Build history of the part. All positions in model axes, mm. Face numbers are marked on the shaded views. A direction names the side the tool comes from. Round coordinates to 2 decimals unless told otherwise and drop trailing zeros. Write each loop counter-clockwise with the first axis right and the second up, starting at its lowest first coordinate (ties: lowest second). Pieces come first, ordered by that corner, then holes. Notation, with made-up numbers: (82.5, -13.75) -> (96.5, -13.75) arc R32 ccw to (96.5, 16.25) -> close; hole circle Ø5 at (23.5, 48). An arc over 180 degrees is marked (long way). Return JSON: item names as keys, results as strings.
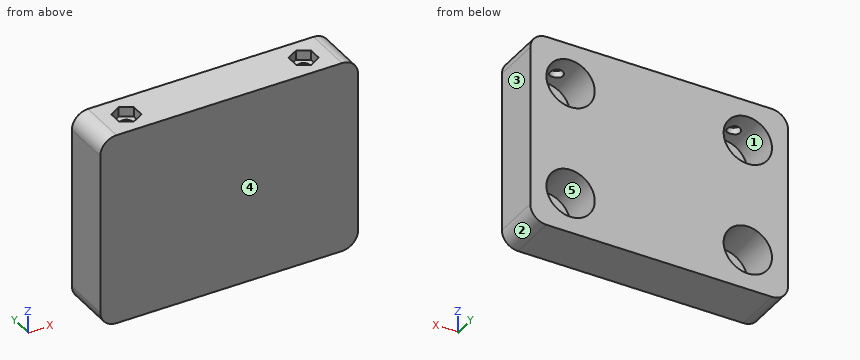
from build123d import *

# Parameters (mm, degrees)
F1_DEPTH = 15
F2_R     = 7.5
F3_DEPTH = 13
F4_R     = 2
F5_DEPTH = 6
F7_DEPTH = 3


with BuildPart() as f1:
    # F0 (on Front) → F1 (new body)
    with BuildSketch(Plane.XZ):
        with BuildLine():
            Line((-0.08701, 32.806785), (-70.08701, 32.806785))
            ThreePointArc((-70.08701, 32.806785), (-73.622544, 31.342318), (-75.08701, 27.806785))
            Line((-75.08701, 27.806785), (-75.08701, -22.193215))
            ThreePointArc((-75.08701, -22.193215), (-73.622544, -25.728749), (-70.08701, -27.193215))
            Line((-70.08701, -27.193215), (-0.08701, -27.193215))
            ThreePointArc((-0.08701, -27.193215), (3.448524, -25.728749), (4.91299, -22.193215))
            Line((4.91299, -22.193215), (4.91299, 27.806785))
            ThreePointArc((4.91299, 27.806785), (3.448524, 31.342318), (-0.08701, 32.806785))
        make_face()
    extrude(amount=F1_DEPTH)

    # F2 (on face) → F3 (cut)
    with BuildSketch(Plane(origin=(0, 0, 0), x_dir=(-1, 0, 0), z_dir=(0, 1, 0))):
        with Locations((7.58701, 20.306785)):
            Circle(F2_R)
        with Locations((62.58701, 20.306785)):
            Circle(F2_R)
        with Locations((62.58701, -14.693215)):
            Circle(F2_R)
        with Locations((7.58701, -14.693215)):
            Circle(F2_R)
    extrude(amount=-F3_DEPTH, mode=Mode.SUBTRACT)

    # F4 (on face) → F5 (cut)
    with BuildSketch(Plane.XY.offset(32.806785)):
        with Locations((-62.58701, -7.5)):
            Circle(F4_R)
        with Locations((-7.58701, -7.5)):
            Circle(F4_R)
    extrude(amount=-F5_DEPTH, mode=Mode.SUBTRACT)

    # F6 (on face) → F7 (cut)
    with BuildSketch(Plane.XY.offset(32.806785)):
        Polygon((-59.08701, -9.520726), (-59.08701, -5.479274), (-62.58701, -3.458548), (-66.08701, -5.479274), (-66.08701, -9.520726), (-62.58701, -11.541452), align=None)
        Polygon((-4.08701, -9.520726), (-4.08701, -5.479274), (-7.58701, -3.458548), (-11.08701, -5.479274), (-11.08701, -9.520726), (-7.58701, -11.541452), align=None)
    extrude(amount=-F7_DEPTH, mode=Mode.SUBTRACT)


solid = f1.part
Q1. Saw through at A-A on y = -7.5. List the corners of the cut face in (x, z).
Verdict:
{"outline": "(-75.09, -22.19) arc R5 ccw to (-70.09, -27.19) -> (-0.09, -27.19) arc R5 ccw to (4.91, -22.19) -> (4.91, 27.81) arc R5 ccw to (-0.09, 32.81) -> (-4.09, 32.81) -> (-4.09, 29.81) -> (-5.59, 29.81) -> (-5.59, 27.54) arc R7.5 cw (long way) to (-9.59, 27.54) -> (-9.59, 29.81) -> (-11.09, 29.81) -> (-11.09, 32.81) -> (-59.09, 32.81) -> (-59.09, 29.81) -> (-60.59, 29.81) -> (-60.59, 27.54) arc R7.5 cw (long way) to (-64.59, 27.54) -> (-64.59, 29.81) -> (-66.09, 29.81) -> (-66.09, 32.81) -> (-70.09, 32.81) arc R5 ccw to (-75.09, 27.81) -> close; hole circle Ø15 at (-62.59, -14.69); hole circle Ø15 at (-7.59, -14.69)"}
Q2. Saw through at B-B on x = -63.5. List the corners of the cut face in (y, z).
Verdict:
{"outline": "(-15, -27.19) -> (0, -27.19) -> (0, -22.14) -> (-13, -22.14) -> (-13, -7.25) -> (0, -7.25) -> (0, 12.86) -> (-13, 12.86) -> (-13, 27.75) -> (-9.28, 27.75) -> (-9.28, 29.81) -> (-11.01, 29.81) -> (-11.01, 32.81) -> (-15, 32.81) -> close; (-5.72, 27.75) -> (0, 27.75) -> (0, 32.81) -> (-3.99, 32.81) -> (-3.99, 29.81) -> (-5.72, 29.81) -> close"}
Q3. 3-axis set-ups, long thin cutter, end or side, ignore diameter. For the marked faces 1 and 2: which of +Z, -Z, +X, -X, +Y, -Y reach the whole face in a straight line?
Verdict:
{"face 1": "+Y", "face 2": "-Z, +X, +Y, -Y"}
Q4. Two-plate mould, pull along X, no slides. Class the marked faces 3, 4 and 5: +X half, -X half, draft (parallel to the pull), parting line (faces both ways), or undercut.
Verdict:
{"face 3": "+X half", "face 4": "draft", "face 5": "undercut"}
Q5. Pin check, flat tips, straight feed: pin 1 Ø0.9 at (y, z) = (-6.5, 31) entering from -X; pin 2 Ø12 at (x, z) = (-6.5, -12.5) entering from +Y; pin 3 Ø1.5 at (y, z) = (-8, 31) entering from +X; pin 4 Ø4.5 at (x, z) = (-65, 22) entering from +Y. Stop position of each tip, or through.
Verdict:
{"pin 1": "stops at x = -74.27", "pin 2": "stops at y = 0", "pin 3": "stops at x = 4.28", "pin 4": "stops at y = -13"}
Q6. Saw through at D-D on z = 25.5. List the corners of the cut face in (x, y), then the cut area to 3 significant figures.
Verdict:
{"outline": "(-75.09, -15) -> (4.91, -15) -> (4.91, 0) -> (-2.18, 0) -> (-2.18, -13) -> (-13, -13) -> (-13, 0) -> (-57.18, 0) -> (-57.18, -13) -> (-68, -13) -> (-68, 0) -> (-75.09, 0) -> close", "area": "919 mm²"}
Q7. Wall check: L1, parallel to Z at x = -65.5, y = -1.5; L2, parallel to X at y = -11, z = -20; L3, parallel to X at y = -7, z = 30.5. Give the ranges that are in metal, low to high.
Verdict:
{"L1": "z = -27.19 to -21.6, -7.78 to 13.4, 27.22 to 32.81", "L2": "x = -75.09 to -67.89, -57.29 to -12.89, -2.29 to 4.91", "L3": "x = -74.3 to -66.09, -59.09 to -11.09, -4.09 to 4.13"}
Q8. Saw through at C-C on x = -14. List the corners of the cut face in (y, z), then the cut area to 3 significant figures.
Verdict:
{"outline": "(-15, -27.19) -> (0, -27.19) -> (0, -18.58) -> (-13, -18.58) -> (-13, -10.8) -> (0, -10.8) -> (0, 16.42) -> (-13, 16.42) -> (-13, 24.2) -> (0, 24.2) -> (0, 32.81) -> (-15, 32.81) -> close", "area": "698 mm²"}
